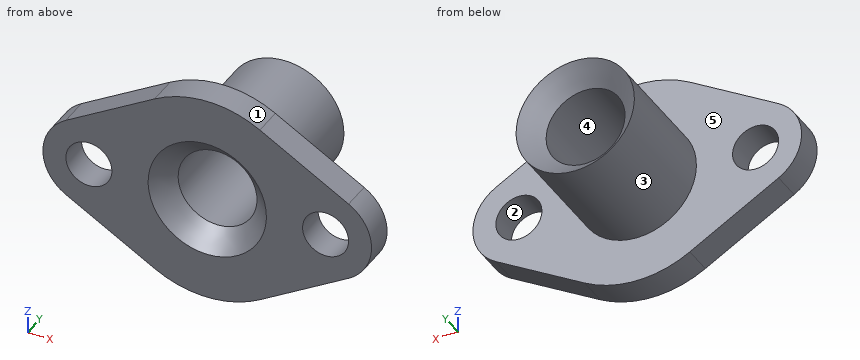
```python
from build123d import *

# Parameters (mm, degrees)
SKETCH_1_R      = 7
SKETCH_1_R_2    = 18
EXTRUDE_1_DEPTH = 9
SKETCH_1_3_R    = 18
SKETCH_1_3_R_2  = 12
EXTRUDE_2_DEPTH = 45
CHAMFER_1_SIZE  = 6


with BuildPart() as part:
    # 草圖1 → 填料-伸長1 (new body)
    with BuildSketch(Plane(origin=(0, 0, 0), x_dir=(1, 0, 0), z_dir=(0, 1, 0))):
        with BuildLine():
            Line((16, -27.712812921), (43, -12.124355653))
            ThreePointArc((43, -12.124355653), (50, 0), (43, 12.124355653))
            Line((43, 12.124355653), (16, 27.712812921))
            ThreePointArc((16, 27.712812921), (0, 32), (-16, 27.712812921))
            Line((-16, 27.712812921), (-43, 12.124355653))
            ThreePointArc((-43, 12.124355653), (-50, 0), (-43, -12.124355653))
            Line((-43, -12.124355653), (-16, -27.712812921))
            ThreePointArc((-16, -27.712812921), (0, -32), (16, -27.712812921))
        make_face()
        with Locations(Location((36, 0, 0), (0, 0, 270))):
            Circle(SKETCH_1_R, mode=Mode.SUBTRACT)
        with Locations(Location((-36, 0, 0), (0, 0, 270))):
            Circle(SKETCH_1_R, mode=Mode.SUBTRACT)
        with Locations(Location((0, 0, 0), (0, 0, 270))):
            Circle(SKETCH_1_R_2, mode=Mode.SUBTRACT)
    extrude(amount=EXTRUDE_1_DEPTH)

    # 草圖1<3> → 填料-伸長2 (add)
    with BuildSketch(Plane(origin=(0, 0, 0), x_dir=(1, 0, 0), z_dir=(0, 1, 0))):
        with Locations(Location((0, 0, 0), (0, 0, 90))):
            Circle(SKETCH_1_3_R)
        with Locations(Location((0, 0, 0), (0, 0, 90))):
            Circle(SKETCH_1_3_R_2, mode=Mode.SUBTRACT)
    extrude(amount=EXTRUDE_2_DEPTH)

    # 導角1
    chamfer_1_edges = [part.edges().sort_by_distance(p)[0] for p in [
        (0, 45, 12),
        (0, 0, 12),
    ]]
    chamfer(chamfer_1_edges, length=CHAMFER_1_SIZE - 0.0001)  # a hair under: the kernel refuses the full size


solid = part.part
```
The listing builds one solid part. Answer for the finished solid, in the listing's coordinates (mm). Face numbers are marked on the shaded views. A direction names the side the tool comes from. Coordinates: 2 decimals unless noted, no trailing zeros. Loops run counter-clockwise (first coordinate to the right, second up) from the corner with the lowest first, then second, coordinate; pieces in that order, holes last. Notation, with made-up numbers: M 17,-30.75 L 57,-30.75 A30 cw 57,-0.75 Z; hole C 7.25,84.25 d6. An arc over 180 degrees is marked long. Answer as a JSON object with one key per item and string values. Group by question number.
Item 1: Section A-A (z = 0) is taken. Give the number of separate pieces and of enclosed holes in the cut face, and give its area (3 significant figures).
Item 2: Which of the six approach directions +Z, -Z, +X, -X, +Y, -Y give full straight-line access (tool end or side, diameter ignored) to the marked faces 4 and 5?
Item 3: Each of these flat-tipped pins is pushed along its axis until it touches: P1, Ø4, axis at x = -25, y = 6, coming from the +Z side; P2, Ø12, axis at x = 23, z = 1, coming from the -Y side; P3, Ø6, axis at x = 2.5, z = 11.5, coming from the -Y side; P4, Ø14.5, axis at x = 0, z = 0, coming from the +Y side. Where does it stop, or does it pass through?
Item 4: Section D-D (y = 25.5) is taken. Write down the section's boundary in (x, z).
Item 5: Section B-B (x = -32.5) is taken. Write down the section's boundary in (y, z).
Item 6: Section C-C (y = 3) is taken. Write down the section's boundary in (x, z).
Item 7: Consider L1, parallel to X at y = 32, z = 0; L2, parallel to Z at x = -2.5, y = 3; L3, parallel to Y at x = -18, z = -5. Determine where each line is inside the solid, lowest interval first.
Item 8: Determine the mould class of the marked faces 1, 2 and 3 for opening direction Z: +Z half, -Z half, draft (parallel to the pull), parting line (faces both ways), or undercut.
Solved:
{
 "1": {"separate pieces": "4", "enclosed holes": "0", "area": "792 mm2"},
 "2": {"face 4": "+Y, -Y", "face 5": "+Y"},
 "3": {"P1": "stops at z = 23.67", "P2": "stops at y = 0", "P3": "stops at y = 3.23", "P4": "passes through"},
 "4": {"outline": "C 0,0 d36; hole C 0,0 d24"},
 "5": {"outline": "M 0,-18.19 L 9,-18.19 L 9,-6.06 L 0,-6.06 Z; M 0,6.06 L 9,6.06 L 9,18.19 L 0,18.19 Z"},
 "6": {"outline": "M -43,-12.12 L -16,-27.71 A32 ccw 16,-27.71 L 43,-12.12 A14 ccw 43,12.12 L 16,27.71 A32 ccw -16,27.71 L -43,12.12 A14 ccw Z; hole C -36,0 d14; hole C 0,0 d30; hole C 36,0 d14"},
 "7": {"L1": "x = -18 to -12, 12 to 18", "L2": "z = -31.9 to -14.79, 14.79 to 31.9", "L3": "y = 0 to 9"},
 "8": {"face 1": "+Z half", "face 2": "undercut", "face 3": "parting line"}
}
